The figure shows three views and two pictorial views of one solid part (mm, origin at its lowest corner). Answer the questions. A direction names the side the tool comes from. Round coordinates to 2 decimals unless told otherwise and drop trailing zeros. Order: outer loops, then holes, each group sorted by start corner. A loop starts at its lowest first (then second) coordinate and runs counter-clockwise, first axis right, second up.
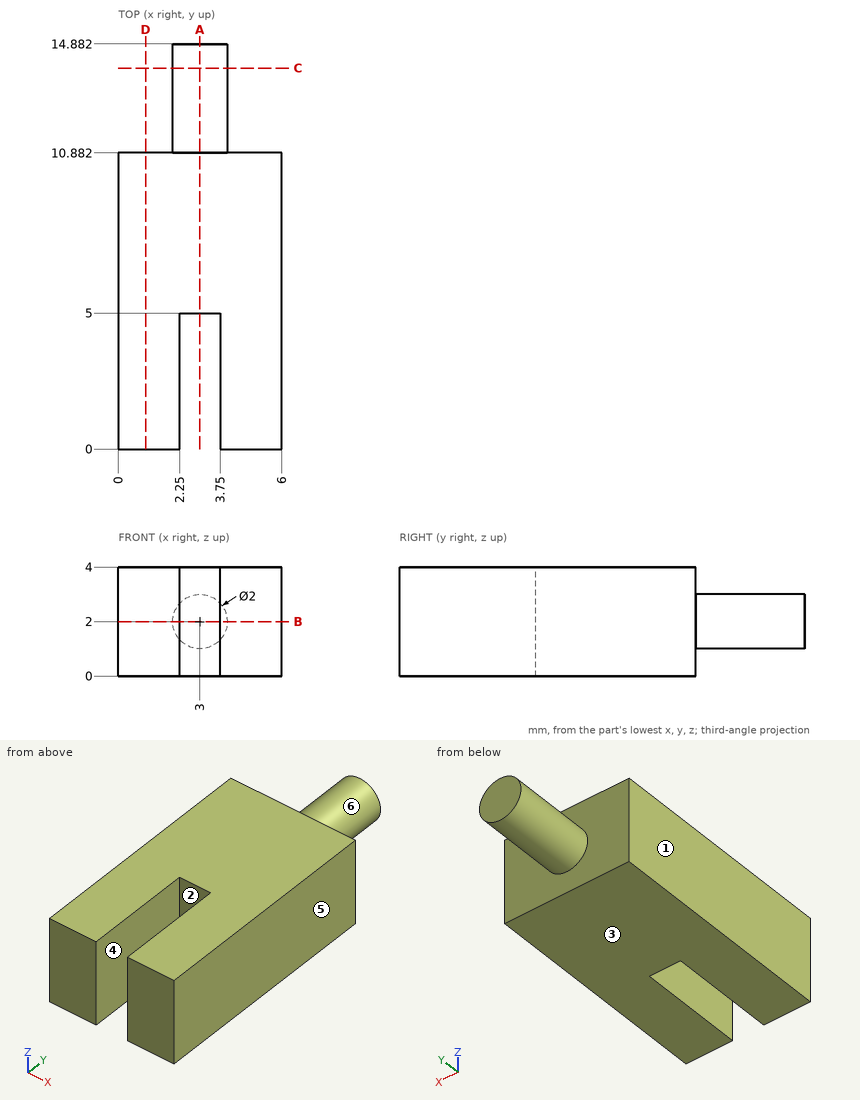
Item 1: Find section B-B (z = 2). Write down the section's boundary in (x, y), plus the area to 3 significant figures.
Item 2: Find section D-D (x = 1). Write down the section's boundary in (y, z).
Item 3: Given pin 1 (2 mm diameter, centred on x = 5.5, z = 2, fed in from -Y), flat-ended and moving along its own axis, determine where the tip first touches the part or whether it passes through.
Item 4: Find section A-A (x = 3). Write down the section's boundary in (y, z), plus the area to 3 significant figures.
Item 5: For a pull along X with two mould halves and no side action, classify the marked faces 1, 2 and 3 as released by +X, released by -X, zero draft, split by the parting line, or undercut.
Item 6: A tool of negligible diameter and unlimited length cuts with its end or side. For the marked faces 4, 5 and 6, from which of +Z, -Z, +X, -X, +Y, -Y can it reach the whole face along a straight path? Write none if from no direction.
Item 7: Find section C-C (y = 14). Write down the section's boundary in (x, z).
Item 8: Find the intervals of material crossed by line 1 along X through (y, z) = (2, 3.7); line 2 along Y through (x, z) = (1.1, 3.5); line 3 along Y through (x, z) = (3.45, 1.85), in increasing order.
Model answer:
1. outline: (0, 0) - (2.25, 0) - (2.25, 5) - (3.75, 5) - (3.75, 0) - (6, 0) - (6, 10.88) - (4, 10.88) - (4, 14.88) - (2, 14.88) - (2, 10.88) - (0, 10.88) - close
1. area: 65.8 mm2
2. outline: (0, 0) - (10.88, 0) - (10.88, 4) - (0, 4) - close
3. pin 1: stops at y = 0
4. outline: (5, 0) - (10.88, 0) - (10.88, 1) - (14.88, 1) - (14.88, 3) - (10.88, 3) - (10.88, 4) - (5, 4) - close
4. area: 31.5 mm2
5. face 1: released by -X
5. face 2: undercut
5. face 3: zero draft
6. face 4: +Z, -Z, -Y
6. face 5: +Z, -Z, +X, +Y, -Y
6. face 6: +Y
7. outline: circle Ø2 at (3, 2)
8. line 1: x = 0 to 2.25, 3.75 to 6
8. line 2: y = 0 to 10.88
8. line 3: y = 5 to 14.88
